The drawing under review shows one solid part. Ordinate dimensions are in mm from its lowest x, y, z. Give positions to 0.01 mm unless a question says otherwise; leave off trailing zeros. Loops run counter-clockwise (first coordinate to the right, second up) from the corner with the lowest first, then second, coordinate; pieces in that order, holes last.
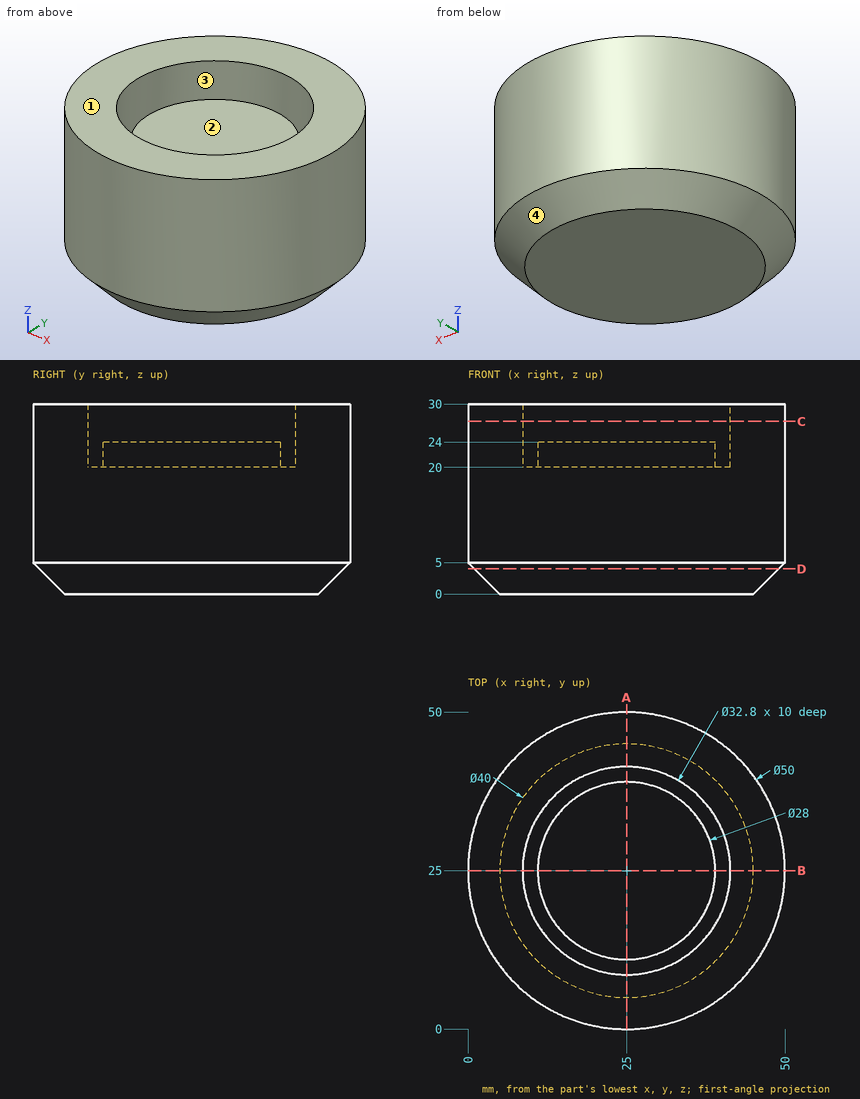
Item 1: Take a section at C-C on z = 27.25. Give the boundary of the cut face in (x, y).
Answer:
outline: circle Ø50 at (25, 25); hole circle Ø32.8 at (25, 25)
Item 2: Take a section at A-A on x = 25. Give the boundary of the cut face in (y, z), and give its area (3 significant figures).
Answer:
outline: (0, 5) - (5, 0) - (45, 0) - (50, 5) - (50, 30) - (41.4, 30) - (41.4, 20) - (39, 20) - (39, 24) - (11, 24) - (11, 20) - (8.6, 20) - (8.6, 30) - (0, 30) - close
area: 1,260 mm2
Item 3: Take a section at D-D on z = 4. Give the boundary of the cut face in (x, y), and give its area (3 significant figures).
Answer:
outline: circle Ø48 at (25, 25)
area: 1,810 mm2
Item 4: For L1, parallel to Y at x = 25, z = 23.75; L2, parallel to Y at x = 25, z = 26.5; L3, parallel to Z at x = 36, y = 17, list the stretches that pass through material, from the lowest coordinate up.
Answer:
L1: y = 0 to 8.6, 11 to 39, 41.4 to 50
L2: y = 0 to 8.6, 41.4 to 50
L3: z = 0 to 24
Item 5: Clearance check with flat-ended pins moving along their axes: pin 1 Ø4 at (x, z) = (21.5, 22) entering from +Y; pin 2 Ø8.5 at (x, y) = (32, 31) entering from +Z; pin 3 Ø5 at (x, z) = (30.5, 12) entering from +Y. State where each tip first meets the part, or that it passes through.
Answer:
pin 1: stops at y = 49.95
pin 2: stops at z = 24
pin 3: stops at y = 49.82
Item 6: The part is to be moulded in two halves that separate along Y. For the marked faces 1, 2, 3 and 4, say which applies: released by +Y, released by -Y, zero draft, split by the parting line, or undercut.
Answer:
face 1: zero draft
face 2: undercut
face 3: undercut
face 4: split by the parting line
